Geometry check sheet. Reference: drawing and pictorial views, mm from the part's lowest x, y, z. A direction names the side the tool comes from. Round coordinates to 2 decimals unless told otherwise and drop trailing zeros. Write each loop counter-clockwise with the first axis right and the second up, starting at its lowest first coordinate (ties: lowest second). Pieces come first, ordered by that corner, then holes. Notation, with made-up numbers: (22.25, 38.25) - (79.25, 38.25) arc R21 cw to (79.25, 61.25) - close; hole circle Ø3 at (-3.5, -4). An arc over 180 degrees is marked (long way). Use one line per item in the form item = value. Start each with the question number.
1) Gauge pin test, flat end, axial feed: P1, Ø1, axis at x = 11.5, z = 2, coming from the +Y side (1 decimal). Record the tip position at first contact, or that the pin passes through.
2) Section check A-A (z = 6.35). Count the separate pieces of the cut face and the enclosed holes in it.
3) Section check D-D (z = 2). Record the boundary of the cut face in (x, y) (1 decimal), then the cut area to 3 significant figures.
4) Section check C-C (y = 6.75). Record the boundary of the cut face in (x, z) (1 decimal).
5) Section check B-B (x = 10). Record the boundary of the cut face in (y, z) (1 decimal), then the cut area to 3 significant figures.
6) Set-up check for the marked faces 1, 2 and 3: record each of +Z, -Z, +X, -X, +Y, -Y from which the full face is reachable in a straight line by a thin tool's end or side.
7) Draft check along Z on the marked faces 4, 5 and 6. Enter one of: +Z half, -Z half, draft (parallel to the pull), parting line (faces both ways), or undercut.
8) Scan line: probe 1 along X at (y, z) = (3.75, 4) (1 decimal). Record every from-to range of solid material in increasing order.
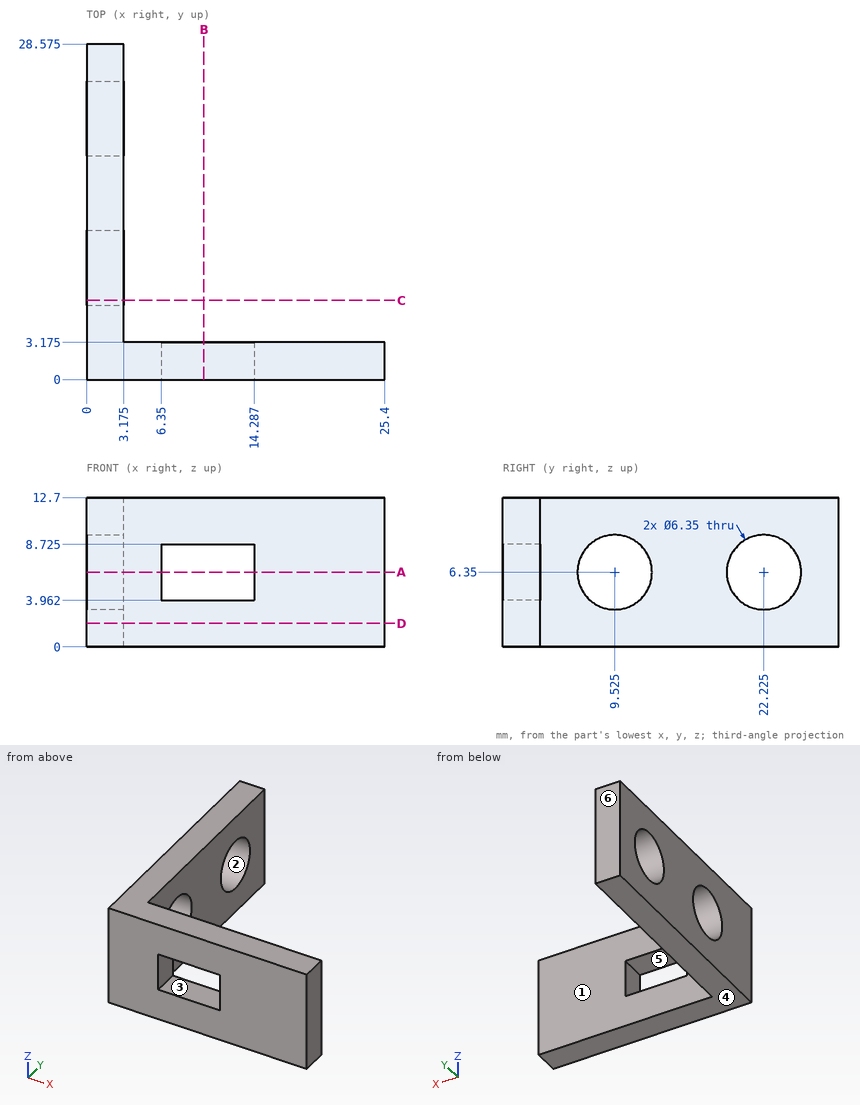
Results are:
q1.P1 = 3.2
q2.separate_pieces = 4
q2.enclosed_holes = 0
q3.outline = (0, 0) - (25.4, 0) - (25.4, 3.2) - (3.2, 3.2) - (3.2, 28.6) - (0, 28.6) - close
q3.area = 161 mm²
q4.outline = (0, 0) - (3.2, 0) - (3.2, 4.8) - (0, 4.8) - close; (0, 7.9) - (3.2, 7.9) - (3.2, 12.7) - (0, 12.7) - close
q5.outline = (0, 0) - (3.2, 0) - (3.2, 4) - (0, 4) - close; (0, 8.7) - (3.2, 8.7) - (3.2, 12.7) - (0, 12.7) - close
q5.area = 25.2 mm²
q6.face_1 = +Z, -Z, +X, +Y
q6.face_2 = +X, -X
q6.face_3 = +Y, -Y
q7.face_4 = -Z half
q7.face_5 = undercut
q7.face_6 = draft
q8.probe_1 = 0 to 3.2
